Could you check a few things on this model? Use its own coordinates, in mm. A direction names the side the tool comes from. Coordinates: 2 decimals unless noted, no trailing zeros. Write each loop counter-clockwise with the first axis right and the second up, starting at its lowest first coordinate (ties: lowest second). Pieces come first, ordered by that corner, then holes.
```python
from build123d import *

# Parameters (mm, degrees)
SKETCH1_R           = 1.5
BOSS_EXTRUDE1_DEPTH = 2
FILLET2_R           = 4
CUT_EXTRUDE1_DEPTH  = 21.099751242
FILLET3_R           = 1


with BuildPart() as part:
    # Sketch1 → Boss-Extrude1 (new body)
    with BuildSketch(Plane(origin=(0, 0, 0), x_dir=(1, 0, 0), z_dir=(0, 1, 0))):
        with BuildLine():
            Line((-9, 10), (-9, 7.937253933))
            ThreePointArc((-9, 7.937253933), (0, -12), (9, 7.937253933))
            Line((9, 7.937253933), (9, 10))
            Line((9, 10), (9, 16))
            Line((9, 16), (-9, 16))
            Line((-9, 16), (-9, 10))
        make_face()
        with Locations(Location((-6, 13, 0), (0, 0, 270))):
            Circle(SKETCH1_R, mode=Mode.SUBTRACT)
        with Locations(Location((6, 13, 0), (0, 0, 270))):
            Circle(SKETCH1_R, mode=Mode.SUBTRACT)
    extrude(amount=BOSS_EXTRUDE1_DEPTH)

    # Fillet2
    fillet2_edges = [part.edges().sort_by_distance(p)[0] for p in [
        (9, 1, -7.937253933),
        (-9, 1, -7.937253933),
        (-9, 1, -16),
        (9, 1, -16),
    ]]
    fillet(fillet2_edges, radius=FILLET2_R)

    # Sketch2 → Cut-Extrude1 (cut, through all)
    with BuildSketch(Plane(origin=(0, 2, 0), x_dir=(1, 0, 0), z_dir=(0, 1, 0))):
        with BuildLine():
            Line((-11.796609682, 2.2), (-9.65, 2.2))
            Line((-9.65, 2.2), (-9.65, 7.255695723))
            ThreePointArc((-9.65, 7.255695723), (-11.151781756, 4.909775878), (-11.796609682, 2.2))
        make_face()
        with BuildLine():
            Line((9.65, 2.2), (9.65, 7.255695723))
            ThreePointArc((9.65, 7.255695723), (11.151781756, 4.909775878), (11.796609682, 2.2))
            Line((11.796609682, 2.2), (9.65, 2.2))
        make_face()
    extrude(amount=-CUT_EXTRUDE1_DEPTH, mode=Mode.SUBTRACT)

    # Fillet3
    fillet3_edges = [part.edges().sort_by_distance(p)[0] for p in [
        (-9.65, 1, -7.141629754),
        (-11.796609682, 1, -2.2),
        (-9.65, 1, -2.2),
        (9.65, 1, -7.141629754),
        (9.65, 1, -2.2),
        (11.796609682, 1, -2.2),
    ]]
    fillet(fillet3_edges, radius=FILLET3_R)


solid = part.part
```
Item 1: If I drill on line 1 along X through (y, z) = (1.15, -13); line 2 along X through (y, z) = (1.9, -14.25); line 3 along Z through (x, y) = (0.25, 1.65), over which ranges is the centre line in solid material (lowest first)?
Item 2: I want a section at C-C, the plane x = 6. List the corners of the cut face in (y, z) for me.
Item 3: Which directions (+Z, -Z, +X, -X, +Y, -Y) give clear straight access to the entire face, cutting with the end or side of a thin tool? Please do faces 1 (the flat face through (0, 1, -16)), 2 (the flat face through (9.65, 1, -5)), 3 (the flat face through (-9.65, 1, -5)).
Item 4: I want a section at A-A, the plane y = 1.55. List the corners of the cut face in (x, z) for me, then the cut area to 3 significant figures.
Item 5: Will these pins go through, and if not, where does the flat tip stop? pin 1 Ø2.5 at (x, z) = (-6, -13) entering from -Y; pin 2 Ø1 at (y, z) = (1.5, -4.5) entering from -X.
Item 6: I want a section at B-B, the plane z = -13.75. List the corners of the cut face in (x, y) for me, then the cut area to 3 significant figures.
Item 7: If we mould it in two halves opening along X, with no side actions, what happens to faces 4 (the cylindrical face through (6.07, 0.99, -14.5)), 5 (the flat face through (0, 2, -2)), 6 (the cylindrical face through (0, 1, 12)), 7 (the cylindrical face through (7.859, 1.014, -14.797))? For each: released by +X, released by -X, zero draft, split by the parting line, or undercut.
Item 8: I want a section at D-D, the plane z = -5.5. List the corners of the cut face in (x, y) for me.
Taken from the geometry:
1. line 1: x = -8.87 to -7.5, -4.5 to 4.5, 7.5 to 8.87
1. line 2: x = -8.31 to -6.83, -5.17 to 5.17, 6.83 to 8.31
1. line 3: z = -16 to 12
2. outline: (0, -15.87) - (2, -15.87) - (2, -14.5) - (0, -14.5) - close; (0, -11.5) - (2, -11.5) - (2, 10.39) - (0, 10.39) - close
3. face 1: -Z, +X, -X, +Y, -Y
3. face 2: -Z, +X, +Y, -Y
3. face 3: -Z, -X, +Y, -Y
4. outline: (-11.93, -1.31) arc R1 ccw to (-10.93, -2.2) - (-10.65, -2.2) arc R1 cw to (-9.65, -3.2) - (-9.65, -6.86) arc R1 ccw to (-9.52, -7.36) arc R4 cw to (-9, -9.33) - (-9, -12) arc R4 ccw to (-5, -16) - (5, -16) arc R4 ccw to (9, -12) - (9, -9.33) arc R4 cw to (9.52, -7.36) arc R1 ccw to (9.65, -6.86) - (9.65, -3.2) arc R1 cw to (10.65, -2.2) - (10.93, -2.2) arc R1 ccw to (11.93, -1.31) arc R12 ccw (long way) to start; hole circle Ø3 at (-6, -13); hole circle Ø3 at (6, -13)
4. area: 514 mm2
5. pin 1: passes through
5. pin 2: stops at x = -9.65
6. outline: (-8.6, 0) - (-7.3, 0) - (-7.3, 2) - (-8.6, 2) - close; (-4.7, 0) - (4.7, 0) - (4.7, 2) - (-4.7, 2) - close; (7.3, 0) - (8.6, 0) - (8.6, 2) - (7.3, 2) - close
6. area: 24.0 mm2
7. face 4: undercut
7. face 5: zero draft
7. face 6: split by the parting line
7. face 7: released by +X
8. outline: (-9.65, 0) - (9.65, 0) - (9.65, 2) - (-9.65, 2) - close
